Model file for the job. Use its own axes, mm. A direction names the side the tool comes from. Round coordinates to 2 decimals unless told otherwise and drop trailing zeros. Order: outer loops, then holes, each group sorted by start corner. A loop starts at its lowest first (then second) coordinate and runs counter-clockwise, first axis right, second up. Notation, with made-up numbers: (14, 45) -> (54, 45) arc R22 ccw to (54, 63) -> close; hole circle Ø10 at (65, 48). An arc over 180 degrees is marked (long way). Use CSV: the item, a comma, the result in double quotes.
Autodesk Inventor part; units mm, degrees
ref_plane "作業平面1" through (230, 0, 0) normal (1, 0, 0) x (0, 1, 0)
ref_plane "作業平面2" through (600, 0, 0) normal (-1, 0, 0) x (0, 0, 1)
ref_plane "作業平面3" through (230, 0, 0) normal (1, 0, 0) x (0, 1, 0)
sketch "スケッチ1" plane through (0, 0, 0) normal (1, 0, 0) x (0, 1, 0)
  line L0 (10, 125) -> (0, 125)
  line L1 (0, 125) -> (0, -125)
  line L2 (0, -125) -> (10, -125)
  line L3 (10, -125) -> (10, 125)
  point P0 (0, 0)
  dimension "d0" = 250
  dimension "d1" = 10
extrude "押し出し1" add sketch "スケッチ1" along normal mid plane 1400
sketch "スケッチ2" plane through (700, 0, 0) normal (1, 0, 0) x (0, 0, -1)
  line L0 (104.6973, 150) -> (-225, 30)
  line L1 (-225, 30) -> (-225, -50)
  line L2 (-225, -50) -> (275, -50)
  line L3 (275, -50) -> (275, 150)
  line L4 (-125, 0) -> (125, 0)
  line L5 (-125, 10) -> (-125, 0)
  line L6 (125, 0) -> (125, 10)
  line L7 (125, 10) -> (-125, 10)
  line L8 (104.6973, 150) -> (275, 150)
  point P0 (0, 0)
  dimension "d4" = 50
  dimension "d5" = 20
  dimension "d6" = 200
  dimension "d7" = 500
  dimension "d8" = 100
  dimension "d9" = 80
extrude "押し出し3" add sketch "スケッチ2" along normal blind 10 contours L8 L3 L2 L1 L0 | L5 L7 L6 L4
ref_plane "作業平面1" through (230, 0, 0) normal (1, 0, 0) x (0, 1, 0)
ref_plane "作業平面2" through (600, 0, 0) normal (-1, 0, 0) x (0, 0, 1)
ref_plane "作業平面3" through (230, 0, 0) normal (1, 0, 0) x (0, 1, 0)
mirror "ミラー3" about plane through (600, 0, 0) normal (-1, 0, 0) of "押し出し3"
sketch "スケッチ4" plane through (230, 0, 0) normal (1, 0, 0) x (0, 1, 0)
  line L0 (40, 205) -> (-30, 205)
  line L1 (-30, 205) -> (-30, -325)
  line L2 (-30, -325) -> (200, -325)
  line L3 (200, -325) -> (200, -72.1281)
  line L4 (200, -72.1281) -> (40, 205)
  line L5 (0, -520.2563) -> (0, 349.2094)
  line L6 (30, 225) -> (-50, 225)
  line L7 (-50, 225) -> (-50, -275)
  line L8 (-50, -275) -> (150, -275)
  point P0 (0, 0)
  dimension "d25" = 230
  dimension "d26" = 20
  dimension "d27" = 20
  dimension "d28" = 50
  dimension "d29" = 30
  dimension "d30" = 70
extrude "押し出し5" add sketch "スケッチ4" along normal blind 10 contours L4 L3 L2 L5 L0 | L5 L8 L1 L0 | L5 L2 L1 L8
sketch "スケッチ5" plane through (700, 0, 0) normal (-1, 0, 0) x (0, 0, 1)
  arc A0 (-199.5342, 116.4458) -> (-65, 20) centre (4.9464, 259.6246) ccw
  arc A1 (-191.3426, 122.1816) -> (-62.1979, 29.5994) centre (4.9464, 259.6246) ccw
  line L0 (-65, 20) -> (-62.1979, 29.5994)
  line L1 (-191.3426, 122.1816) -> (-199.5342, 116.4458)
  line L2 (125, 10) -> (-125, 10)
  line L3 (-125, 10) -> (-125, 0)
  line L4 (-125, 10) -> (-199.5342, 116.4458)
  point P0 (0, 0)
  dimension "d33" = 10
  dimension "d36" = 10
  dimension "d37" = 60
  dimension "d42" = 125
extrude "押し出し6" add sketch "スケッチ5" along normal up to next
mirror "ミラー5" about plane through (0, 0, 0) normal (1, 0, 0) of "押し出し5", "押し出し3", "ミラー3", "押し出し6"
properties part number "F-wing"
Q1. Pin check, flat tips, straight feed: pin 1 (11 mm diameter, centred on x = 105.5, y = 3.5, fed in from -Z); pin 2 (2 mm diameter, centred on x = 514.5, z = 106, fed in from -Y); pin 3 (8 mm diameter, centred on x = 706.5, y = 7.5, fed in from -Z). Stop position of each tip, or through.
From the geometry:
pin 1,"stops at z = -125"
pin 2,"stops at y = 0"
pin 3,"stops at z = -275"
Q2. Which spindle directions (+Z, -Z, +X, -X, +Y, -Y) get a long thin tool onto all of the face, cutting with end or side? Do faces 1 (the flat face through (-495.07, 90.84, 57.84)), 2 (the flat face through (-367, 0, 2)), 3 (the flat face through (-700, 51, -84)). Say none if no direction does.
From the geometry:
face 1,"+Z, -X, +Y"
face 2,"+Z, -Z, -Y"
face 3,"none"
Q3. Cut at B-B (y = 162.5). Give the cut face in (x, z), plus the area to 3 significant figures.
From the geometry:
outline,"(-240, -325) -> (-230, -325) -> (-230, -7.18) -> (-240, -7.18) -> close; (230, -325) -> (240, -325) -> (240, -7.18) -> (230, -7.18) -> close"
area,"6,360 mm²"
Q4. Mould opens along Y. For faces 4 (the cylindrical face through (-601.4, 57.437, -141.453)), 5 (the flat face through (704.93, 90.84, 57.84)), 6 (the flat face through (-3, 0, 2)) say: +Y half, -Y half, draft (parallel to the pull), parting line (faces both ways), or undercut.
From the geometry:
face 4,"undercut"
face 5,"+Y half"
face 6,"-Y half"
Q5. Cut at A-A (z = -238.5). Give the cut face in (x, y), plus the area to 3 significant figures.
From the geometry:
outline,"(-710, -50) -> (-700, -50) -> (-700, 150) -> (-710, 150) -> close; (-500, -50) -> (-490, -50) -> (-490, 150) -> (-500, 150) -> close; (-240, -30) -> (-230, -30) -> (-230, 200) -> (-240, 200) -> close; (230, -30) -> (240, -30) -> (240, 200) -> (230, 200) -> close; (490, -50) -> (500, -50) -> (500, 150) -> (490, 150) -> close; (700, -50) -> (710, -50) -> (710, 150) -> (700, 150) -> close"
area,"12,600 mm²"
Q6. Cut at D-D (z = -146). State how many separate pieces and enclosed holes the cut face has, plus the area to 3 significant figures.
From the geometry:
separate pieces,"4"
enclosed holes,"0"
area,"17,700 mm²"
Q7. Cut at C-C (x = 548.5). Give the cut face in (y, z).
From the geometry:
outline,"(0, -125) -> (10, -125) -> (10, 125) -> (0, 125) -> close; (20, -65) arc R249.62 ccw to (116.45, -199.53) -> (122.18, -191.34) arc R239.62 cw to (29.6, -62.2) -> close"
Q8. Probe line 1 along X through (y, z) = (58.5, 64); line 2 along X through (y, z) = (89, 107); line 3 along X through (y, z) = (-38.5, -161). List the from-to ranges inside material, lowest first.
From the geometry:
line 1,"x = -710 to -700, -500 to -490, -240 to -230, 230 to 240, 490 to 500, 700 to 710"
line 2,"x = -240 to -230, 230 to 240"
line 3,"x = -710 to -700, -500 to -490, 490 to 500, 700 to 710"
